from build123d import *

# Parameters (mm, degrees)
BOSS_EXTRUDE2_DEPTH   = 14
CUT_EXTRUDE1_START    = -10
CUT_EXTRUDE1_DEPTH    = 93.322536556
BOSS_EXTRUDE3_DEPTH   = 2
FILLET6_R             = 8
SKETCH7_W             = 0.005
SKETCH7_H             = 82
CUT_EXTRUDE3_DEPTH    = 83.686153771
BOSS_EXTRUDE4_DEPTH   = 8
BOSS_EXTRUDE5_START   = -2
SKETCH12_W            = 8.228592419
SKETCH12_H            = 4.95
BOSS_EXTRUDE5_DEPTH   = 10
SKETCH9_R             = 1.5
CUT_EXTRUDE4_DEPTH    = 87.029065006
BOSS_EXTRUDE6_DEPTH   = 8
BOSS_EXTRUDE15_START  = -2
SKETCH15_W            = 7.945
SKETCH15_H            = 4.95
BOSS_EXTRUDE15_DEPTH  = 10
SKETCH16_R            = 1.5
CUT_EXTRUDE5_DEPTH    = 87.029065006
FILLET9_R             = 5
FILLET10_R            = 5
FILLET11_R            = 5
FILLET12_R            = 5
FILLET13_R            = 5
BOSS_EXTRUDE16_START  = -4
BOSS_EXTRUDE16_DEPTH  = 10
SKETCH18_R            = 4
CUT_EXTRUDE6_DEPTH    = 93.915997839
SKETCH19_W            = 20
SKETCH19_H            = 10
BOSS_EXTRUDE17_DEPTH  = 15
SKETCH20_R            = 4
CUT_EXTRUDE7_DEPTH    = 93.915997839
FILLET14_R            = 5
CUT_EXTRUDE9_START    = -5.282098
SKETCH21_W            = 8
SKETCH21_H            = 12
CUT_EXTRUDE9_DEPTH    = 5.282098
CROQUIS1_W            = 114.881967112
CROQUIS1_H            = 161.64199769
CORTAR_EXTRUIR2_DEPTH = 4.95
CROQUIS2_W            = 88.205530212
CROQUIS2_H            = 82
CORTAR_EXTRUIR3_DEPTH = 51.95


with BuildPart() as part:
    # Sketch1 → Boss-Extrude2 (new body)
    with BuildSketch(Plane(origin=(0, 0, 0), x_dir=(1, 0, 0), z_dir=(0, 1, 0))):
        with BuildLine():
            Line((0, 41), (-47, 41))
            Line((-47, 41), (-47, -41))
            Line((-47, -41), (0, -41))
            add(Edge.make_bspline(
                [(0, -41), (70, -41), (70, 0), (70, 41), (0, 41)],
                knots=[4.71238898, 4.71238898, 4.71238898, 6.283185307, 6.283185307, 7.853981634, 7.853981634, 7.853981634], degree=2, weights=[1, 0.707106781, 1, 0.707106781, 1]))
        make_face()
    extrude(amount=BOSS_EXTRUDE2_DEPTH)

    # Sketch3 → Cut-Extrude1 (cut, through all)
    with BuildSketch(Plane(origin=(0, 14, 0), x_dir=(1, 0, 0), z_dir=(0, 1, 0)).offset(CUT_EXTRUDE1_START)):
        with BuildLine():
            Line((0, 36), (-42, 36))
            Line((-42, 36), (-42, -36))
            Line((-42, -36), (0, -36))
            add(Edge.make_bspline(
                [(0, -36), (65, -36), (65, 0), (65, 36), (0, 36)],
                knots=[4.71238898, 4.71238898, 4.71238898, 6.283185307, 6.283185307, 7.853981634, 7.853981634, 7.853981634], degree=2, weights=[1, 0.707106781, 1, 0.707106781, 1]))
        make_face()
    extrude(amount=CUT_EXTRUDE1_DEPTH, mode=Mode.SUBTRACT)

    # Sketch5 → Boss-Extrude3 (add)
    with BuildSketch(Plane(origin=(0, 14, 0), x_dir=(1, 0, 0), z_dir=(0, 1, 0))):
        with BuildLine():
            Line((-47, 41), (-47, -41))
            Line((-47, -41), (0, -41))
            add(Edge.make_bspline(
                [(0, -41), (70, -41), (70, 0), (70, 41), (0, 41)],
                knots=[4.71238898, 4.71238898, 4.71238898, 6.283185307, 6.283185307, 7.853981634, 7.853981634, 7.853981634], degree=2, weights=[1, 0.707106781, 1, 0.707106781, 1]))
            Line((0, 41), (-47, 41))
        make_face()
        with BuildLine():
            Line((8.5, 27.5), (-6.016685226, 27.5))
            ThreePointArc((-6.016685226, 27.5), (-42, 0), (-6.016685226, -27.5))
            Line((-6.016685226, -27.5), (8.5, -27.5))
            add(Edge.make_bspline(
                [(8.5, -27.5), (58.152777778, -27.5), (58.152777778, 0), (58.152777778, 27.5), (8.5, 27.5)],
                knots=[1.570796327, 1.570796327, 1.570796327, 3.141592654, 3.141592654, 4.71238898, 4.71238898, 4.71238898], degree=2, weights=[1, 0.707106781, 1, 0.707106781, 1]))
        make_face(mode=Mode.SUBTRACT)
    extrude(amount=BOSS_EXTRUDE3_DEPTH)

    # Fillet6
    fillet6_edges = [part.edges().sort_by_distance(p)[0] for p in [
        (-21, 14, 36),
        (65, 14, 0),
        (-21, 14, -36),
    ]]
    fillet(fillet6_edges, radius=FILLET6_R)

    # Sketch7 → Cut-Extrude3 (cut, through all)
    with BuildSketch(Plane(origin=(0, 16, 0), x_dir=(1, 0, 0), z_dir=(0, 1, 0))):
        with Locations((-0.0025, 0)):
            Rectangle(SKETCH7_W, SKETCH7_H)
    extrude(amount=-CUT_EXTRUDE3_DEPTH, mode=Mode.SUBTRACT)


with BuildPart() as cut_extrude3_piece_1:
    # of the separate pieces the step leaves, piece 1, a body of its own (cut_extrude3_pieces)
    add(part.part.solids().sort_by_distance((0, 6, -36))[0])

    # Sketch12 → Boss-Extrude5 (add)
    with BuildSketch(Plane.XY.offset(41).offset(BOSS_EXTRUDE5_START)):
        with Locations((4.114296209, 2.475)):
            Rectangle(SKETCH12_W, SKETCH12_H)
    extrude(amount=BOSS_EXTRUDE5_DEPTH)


with BuildPart() as cut_extrude3_piece_2:
    # of the separate pieces the step leaves, piece 2, a body of its own (cut_extrude3_pieces)
    add(part.part.solids().sort_by_distance((-42, 14, -28))[0])

    # Sketch8 → Boss-Extrude4 (add)
    with BuildSketch(Plane.XY.offset(41)):
        Polygon((-8.005, 0), (-0.005, 0), (-0.005, 5), (8.228592419, 5), (8.228592419, 10), (0, 10), (-8.005, 10), align=None)
    extrude(amount=BOSS_EXTRUDE4_DEPTH)


with BuildPart() as cut_extrude4_tool:
    # Sketch9 → Cut-Extrude4 (new, through all)
    with BuildSketch(Plane(origin=(0, 10, 0), x_dir=(1, 0, 0), z_dir=(0, 1, 0))):
        with Locations(Location((4.228592419, -45, 0), (0, 0, 270))):
            Circle(SKETCH9_R)
    extrude(amount=-CUT_EXTRUDE4_DEPTH)


with BuildPart() as cut_extrude3_piece_1_1:
    add(cut_extrude3_piece_1.part)

    # Cut-Extrude4: cut by cut_extrude4_tool
    add(cut_extrude4_tool.part, mode=Mode.SUBTRACT)

    # Sketch15 → Boss-Extrude15 (add)
    with BuildSketch(Plane(origin=(0, 0, -41), x_dir=(-1, 0, 0), z_dir=(0, 0, -1)).offset(BOSS_EXTRUDE15_START)):
        with Locations((-4.0225, 2.475)):
            Rectangle(SKETCH15_W, SKETCH15_H)
    extrude(amount=BOSS_EXTRUDE15_DEPTH)


with BuildPart() as cut_extrude3_piece_2_1:
    add(cut_extrude3_piece_2.part)

    # Cut-Extrude4: cut by cut_extrude4_tool
    add(cut_extrude4_tool.part, mode=Mode.SUBTRACT)

    # Sketch14 → Boss-Extrude6 (add)
    with BuildSketch(Plane(origin=(0, 0, -41), x_dir=(-1, 0, 0), z_dir=(0, 0, -1))):
        Polygon((8.005, 0), (0, 0), (0, 5), (-7.995, 5), (-7.995, 10), (8.005, 10), align=None)
    extrude(amount=BOSS_EXTRUDE6_DEPTH)


with BuildPart() as cut_extrude5_tool:
    # Sketch16 → Cut-Extrude5 (new, through all)
    with BuildSketch(Plane(origin=(0, 10, 0), x_dir=(1, 0, 0), z_dir=(0, 1, 0))):
        with Locations(Location((3.995, 45, 0), (0, 0, 180))):
            Circle(SKETCH16_R)
    extrude(amount=-CUT_EXTRUDE5_DEPTH)


with BuildPart() as cut_extrude3_piece_1_2:
    add(cut_extrude3_piece_1_1.part)

    # Cut-Extrude5: cut by cut_extrude5_tool
    add(cut_extrude5_tool.part, mode=Mode.SUBTRACT)

    # Fillet10
    fillet10_edges = [cut_extrude3_piece_1_2.edges().sort_by_distance(p)[0] for p in [
        (7.995, 2.475, -49),
    ]]
    fillet(fillet10_edges, radius=FILLET10_R)

    # Fillet13
    fillet13_edges = [cut_extrude3_piece_1_2.edges().sort_by_distance(p)[0] for p in [
        (8.228592419, 2.475, 49),
    ]]
    fillet(fillet13_edges, radius=FILLET13_R)

    # Sketch13 → Boss-Extrude16 (add)
    with BuildSketch(Plane(origin=(0, 4, 0), x_dir=(1, 0, 0), z_dir=(0, 1, 0)).offset(BOSS_EXTRUDE16_START)):
        with BuildLine():
            Line((77.862579899, -17.449607958), (68.480918968, 8.495153988))
            add(Edge.make_bspline(
                [(25.721063073, -38.131875474), (80.737725462, -25.400755175), (68.480918968, 8.495153988)],
                knots=[5.088647992, 5.088647992, 5.088647992, 6.491896136, 6.491896136, 6.491896136], degree=2, weights=[1, 0.763794923, 1]))
            Line((25.721063073, -38.131875474), (72.500386182, -27.306915105))
            ThreePointArc((72.500386182, -27.306915105), (77.397822901, -23.583909635), (77.862579899, -17.449607958))
        make_face()
    extrude(amount=BOSS_EXTRUDE16_DEPTH)

    # Sketch18 → Cut-Extrude6 (cut, through all)
    with BuildSketch(Plane(origin=(0, 10, 0), x_dir=(1, 0, 0), z_dir=(0, 1, 0))):
        with Locations(Location((70.809530882, -20, 0), (0, 0, 270))):
            Circle(SKETCH18_R)
    extrude(amount=-CUT_EXTRUDE6_DEPTH, mode=Mode.SUBTRACT)

    # Croquis1 → Cortar-Extruir2 (cut)
    with BuildSketch(Plane(origin=(0, 0, 0), x_dir=(-1, 0, 0), z_dir=(0, -1, 0))):
        with Locations((-57.440983556, 31.820998845)):
            Rectangle(CROQUIS1_W, CROQUIS1_H)
    extrude(amount=-CORTAR_EXTRUIR2_DEPTH, mode=Mode.SUBTRACT)

    # Croquis2 → Cortar-Extruir3 (cut)
    with BuildSketch(Plane(origin=(0, 4.95, 0), x_dir=(-1, 0, 0), z_dir=(0, -1, 0))):
        with Locations((-44.102765106, 0)):
            Rectangle(CROQUIS2_W, CROQUIS2_H)
    extrude(amount=-CORTAR_EXTRUIR3_DEPTH, mode=Mode.SUBTRACT)


with BuildPart() as cut_extrude3_piece_2_2:
    add(cut_extrude3_piece_2_1.part)

    # Cut-Extrude5: cut by cut_extrude5_tool
    add(cut_extrude5_tool.part, mode=Mode.SUBTRACT)

    # Fillet9
    fillet9_edges = [cut_extrude3_piece_2_2.edges().sort_by_distance(p)[0] for p in [
        (7.995, 7.5, -49),
    ]]
    fillet(fillet9_edges, radius=FILLET9_R)

    # Fillet11
    fillet11_edges = [cut_extrude3_piece_2_2.edges().sort_by_distance(p)[0] for p in [
        (-8.005, 5, -49),
    ]]
    fillet(fillet11_edges, radius=FILLET11_R)

    # Fillet12
    fillet12_edges = [cut_extrude3_piece_2_2.edges().sort_by_distance(p)[0] for p in [
        (-8.005, 5, 49),
        (8.228592419, 7.5, 49),
    ]]
    fillet(fillet12_edges, radius=FILLET12_R)

    # Sketch19 → Boss-Extrude17 (add)
    with BuildSketch(Plane.ZY.offset(47)):
        with Locations((20, 5)):
            Rectangle(SKETCH19_W, SKETCH19_H)
    extrude(amount=BOSS_EXTRUDE17_DEPTH)

    # Sketch20 → Cut-Extrude7 (cut, through all)
    with BuildSketch(Plane(origin=(0, 10, 0), x_dir=(1, 0, 0), z_dir=(0, 1, 0))):
        with Locations(Location((-55, -20, 0), (0, 0, 270))):
            Circle(SKETCH20_R)
    extrude(amount=-CUT_EXTRUDE7_DEPTH, mode=Mode.SUBTRACT)

    # Fillet14
    fillet14_edges = [cut_extrude3_piece_2_2.edges().sort_by_distance(p)[0] for p in [
        (-62, 5, 10),
        (-62, 5, 30),
    ]]
    fillet(fillet14_edges, radius=FILLET14_R)

    # Sketch21 → Cut-Extrude9 (cut)
    with BuildSketch(Plane.ZY.offset(47).offset(CUT_EXTRUDE9_START)):
        with Locations((0, 10)):
            Rectangle(SKETCH21_W, SKETCH21_H)
    extrude(amount=CUT_EXTRUDE9_DEPTH, mode=Mode.SUBTRACT)


solid = cut_extrude3_piece_2_2.part
Can you work these out from the model? Positions are in its coordinate system, mm. A direction names the side the tool comes from. Coordinates: 2 decimals unless noted, no trailing zeros. Loops run counter-clockwise (first coordinate to the right, second up) from the corner with the lowest first, then second, coordinate; pieces in that order, holes last. Notation, with made-up numbers: (86.5, -14.75) - (121.5, -14.75) arc R22 ccw to (121.5, 8.25) - close; hole circle Ø9 at (-37.75, 28). An arc over 180 degrees is marked (long way). Put each result on its own line as item: value. Start each with the question number.
Item 1: Suppose I cut it at D-D (x = 1). Please give me the cut outline in (y, z).
Item 2: Suppose I cut it at B-B (y = 1). Please give me the cut outline in (x, z) (3 decimals).
Item 3: Suppose I cut it at A-A (x = -55). Please give me the cut outline in (y, z), and give its area (3 significant figures).
Item 4: If we mould it in two halves opening along Y, with no side actions, what happens to faces 5 (the face through (-42, 9, 20)), 6 (the face through (0, 10, 45)), 7 (the face through (-62, 5, 20))? For each: +Y half, -Y half, draft (parallel to the pull), parting line (faces both ways), or undercut.
Item 5: If I drill on line 1 along X through (y, z) = (6.75, 20); line 2 along Z through (x, y) = (-42.5, 12.25); line 3 along Y through (x, z) = (-7.5, 25), over which ranges is the centre line in solid material (lowest first)?
Item 6: Suppose I cut it at C-C (z = 45). Please give me the cut outline in (x, y) (3 decimals).
Item 7: Which directions (+Z, -Z, +X, -X, +Y, -Y) give clear straight access to the entire face, cutting with the end or side of a thin tool? Please do faces 1 (the face through (-51, 10, 18)), 2 (the face through (-28.886, 14.986, -23.99)), 3 (the face through (0, 10, -45)), 4 (the face through (-3, 15, 27.5)).
Item 8: For pin 1 (6.5 mm diameter, centred on x = -3, z = 46, fed in from +Y); pin 2 (5 mm diameter, centred on y = 9.5, z = -25, fed in from +X); pin 3 (8 mm diameter, centred on x = -25.5, y = 4.5, fed in from -Z); pin 4 (1.8 mm diameter, centred on x = 4.23, z = 45, fed in from -Y), each with a flat end and sliding along its axis, tell me the tip position at first contact or that it passes through.
Here are the results:
1. outline: (5, -49) - (10, -49) - (10, -41) - (5, -41) - close; (5, 41) - (10, 41) - (10, 49) - (5, 49) - close
2. outline: (-62, 15) arc R5 ccw to (-57, 10) - (-47, 10) - (-47, -41) - (-8.005, -41) - (-8.005, -44) arc R5 ccw to (-3.005, -49) - (0, -49) - (0, -41) - (-0.005, -41) - (-0.005, 49) - (-3.005, 49) arc R5 ccw to (-8.005, 44) - (-8.005, 41) - (-47, 41) - (-47, 30) - (-57, 30) arc R5 ccw to (-62, 25) - close; hole circle Ø8 at (-55, 20)
3. outline: (0, 10) - (10, 10) - (10, 16) - (0, 16) - close; (0, 24) - (10, 24) - (10, 30) - (0, 30) - close
3. area: 120 mm²
4. face 5: undercut
4. face 6: +Y half
4. face 7: draft
5. line 1: -62 to -59, -51 to -42
5. line 2: -41 to -4, 4 to 41
5. line 3: 0 to 4
6. outline: (-7.904, 0) - (-0.005, 0) - (-0.005, 5) - (2.729, 5) - (2.729, 10) - (-7.904, 10) - close; (5.729, 5) - (8.128, 5) - (8.128, 10) - (5.729, 10) - close
7. face 1: +Z, -Z, -X, +Y
7. face 2: +Y
7. face 3: -Z, +X, -X, +Y
7. face 4: +X, +Y
8. pin 1: y = 10
8. pin 2: x = -42
8. pin 3: z = -41
8. pin 4: through
